from build123d import *

# Parameters (mm, degrees)
SKETCH1_W                                    = 107.95
SKETCH1_H                                    = 127
EXTRUDE1_DEPTH                               = 9.525
CBORE_FOR_M5_HEX_HEAD_CAP_SCREW2_D           = 5.5
CBORE_FOR_M5_HEX_HEAD_CAP_SCREW2_CBORE_D     = 12.24
CBORE_FOR_M5_HEX_HEAD_CAP_SCREW2_CBORE_DEPTH = 3.65
LPATTERN5_COUNT                              = 3
LPATTERN5_PITCH                              = 25.4
LPATTERN6_COUNT                              = 2
LPATTERN6_PITCH                              = 88.9
LPATTERN6_COPY_1_D                           = 5.5
LPATTERN6_COPY_1_CBORE_D                     = 12.24
LPATTERN6_COPY_1_CBORE_DEPTH                 = 3.65
LPATTERN6_COPY_2_D                           = 5.5
LPATTERN6_COPY_2_CBORE_D                     = 12.24
LPATTERN6_COPY_2_CBORE_DEPTH                 = 3.65
M5X0_8_TAPPED_HOLE1_D                        = 4.2
LPATTERN7_COUNT                              = 5
LPATTERN7_PITCH                              = 25.4
LPATTERN8_COUNT                              = 2
LPATTERN8_PITCH                              = 63.5
LPATTERN8_COPY_1_D                           = 4.2
LPATTERN8_COPY_2_D                           = 4.2
LPATTERN8_COPY_3_D                           = 4.2
LPATTERN8_COPY_4_D                           = 4.2
SKETCH16_W                                   = 107.95
SKETCH16_H                                   = 57.15
EXTRUDE2_DEPTH                               = 3.175


with BuildPart() as part:
    # Sketch1 → Extrude1 (new body)
    with BuildSketch(Plane.XY):
        Rectangle(SKETCH1_W, SKETCH1_H)
    extrude(amount=EXTRUDE1_DEPTH)

    # CBORE for M5 Hex Head Cap Screw2 (through all)
    with Locations(Plane(origin=(-44.45, -50.8, 9.525), x_dir=(1, 0, 0), z_dir=(0, 0, 1))):
        with Locations((0, 0)):
            cbore_for_m5_hex_head_cap_screw2 = CounterBoreHole(CBORE_FOR_M5_HEX_HEAD_CAP_SCREW2_D / 2, CBORE_FOR_M5_HEX_HEAD_CAP_SCREW2_CBORE_D / 2, CBORE_FOR_M5_HEX_HEAD_CAP_SCREW2_CBORE_DEPTH)

    # LPattern5: CBORE for M5 Hex Head Cap Screw2 ×3
    with Locations(*[(0, i * LPATTERN5_PITCH, 0) for i in range(1, LPATTERN5_COUNT)]):
        add(cbore_for_m5_hex_head_cap_screw2, mode=Mode.SUBTRACT)

    # LPattern6: CBORE for M5 Hex Head Cap Screw2 ×2
    with Locations(*[(i * LPATTERN6_PITCH, 0, 0) for i in range(1, LPATTERN6_COUNT)]):
        add(cbore_for_m5_hex_head_cap_screw2, mode=Mode.SUBTRACT)

    # LPattern6 copy 1 (through all)
    with Locations(Plane(origin=(44.45, -25.4, 9.525), x_dir=(1, 0, 0), z_dir=(0, 0, 1))):
        with Locations((0, 0)):
            CounterBoreHole(LPATTERN6_COPY_1_D / 2, LPATTERN6_COPY_1_CBORE_D / 2, LPATTERN6_COPY_1_CBORE_DEPTH)

    # LPattern6 copy 2 (through all)
    with Locations(Plane(origin=(44.45, 0, 9.525), x_dir=(1, 0, 0), z_dir=(0, 0, 1))):
        with Locations((0, 0)):
            CounterBoreHole(LPATTERN6_COPY_2_D / 2, LPATTERN6_COPY_2_CBORE_D / 2, LPATTERN6_COPY_2_CBORE_DEPTH)

    # M5x0.8 Tapped Hole1 (through all)
    with Locations(Plane(origin=(-31.75, -50.8, 9.525), x_dir=(1, 0, 0), z_dir=(0, 0, 1))):
        with Locations((0, 0)):
            m5x0_8_tapped_hole1 = Hole(M5X0_8_TAPPED_HOLE1_D / 2)

    # LPattern7: M5x0.8 Tapped Hole1 ×5
    with Locations(*[(0, i * LPATTERN7_PITCH, 0) for i in range(1, LPATTERN7_COUNT)]):
        add(m5x0_8_tapped_hole1, mode=Mode.SUBTRACT)

    # LPattern8: M5x0.8 Tapped Hole1 ×2
    with Locations(*[(i * LPATTERN8_PITCH, 0, 0) for i in range(1, LPATTERN8_COUNT)]):
        add(m5x0_8_tapped_hole1, mode=Mode.SUBTRACT)

    # LPattern8 copy 1 (through all)
    with Locations(Plane(origin=(31.75, -25.4, 9.525), x_dir=(1, 0, 0), z_dir=(0, 0, 1))):
        with Locations((0, 0)):
            Hole(LPATTERN8_COPY_1_D / 2)

    # LPattern8 copy 2 (through all)
    with Locations(Plane(origin=(31.75, 0, 9.525), x_dir=(1, 0, 0), z_dir=(0, 0, 1))):
        with Locations((0, 0)):
            Hole(LPATTERN8_COPY_2_D / 2)

    # LPattern8 copy 3 (through all)
    with Locations(Plane(origin=(31.75, 25.4, 9.525), x_dir=(1, 0, 0), z_dir=(0, 0, 1))):
        with Locations((0, 0)):
            Hole(LPATTERN8_COPY_3_D / 2)

    # LPattern8 copy 4 (through all)
    with Locations(Plane(origin=(31.75, 50.8, 9.525), x_dir=(1, 0, 0), z_dir=(0, 0, 1))):
        with Locations((0, 0)):
            Hole(LPATTERN8_COPY_4_D / 2)

    # Sketch16 → Extrude2 (cut)
    with BuildSketch(Plane(origin=(0, 0, 0), x_dir=(-1, 0, 0), z_dir=(0, 0, -1))):
        with Locations((0, 34.925)):
            Rectangle(SKETCH16_W, SKETCH16_H)
    extrude(amount=-EXTRUDE2_DEPTH, mode=Mode.SUBTRACT)


solid = part.part
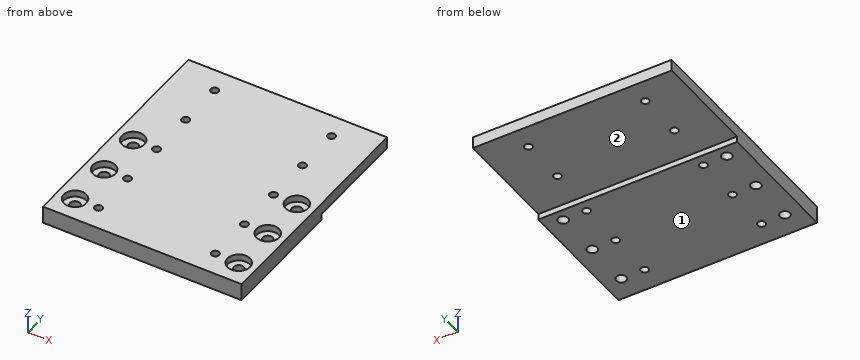
Read the model definition and answer for the solid it produces. Units are mm, in the model's axes. Face numbers are marked on the shaded views. A direction names the side the tool comes from. Coordinates: 2 decimals unless noted, no trailing zeros. Loops run counter-clockwise (first coordinate to the right, second up) from the corner with the lowest first, then second, coordinate; pieces in that order, holes last. Notation, with made-up numbers: (-32, 75) -> (-5, 75) arc R21 cw to (-5, 97) -> close; hole circle Ø9 at (75, -6.5). An arc over 180 degrees is marked (long way). Answer in a Markdown table with one row per item.
Item 1: A cutting plane is placed at B-B on y = 0. Determine the outline of the cut face in (x, z) (3 decimals).
Returned:
| item | result |
|---|---|
| outline | (-53.975, 0) -> (-47.2, 0) -> (-47.2, 5.875) -> (-50.57, 5.875) -> (-50.57, 9.525) -> (-53.975, 9.525) -> close; (-41.7, 0) -> (-33.85, 0) -> (-33.85, 9.525) -> (-38.33, 9.525) -> (-38.33, 5.875) -> (-41.7, 5.875) -> close; (-29.65, 0) -> (29.65, 0) -> (29.65, 9.525) -> (-29.65, 9.525) -> close; (33.85, 0) -> (41.7, 0) -> (41.7, 5.875) -> (38.33, 5.875) -> (38.33, 9.525) -> (33.85, 9.525) -> close; (47.2, 0) -> (53.975, 0) -> (53.975, 9.525) -> (50.57, 9.525) -> (50.57, 5.875) -> (47.2, 5.875) -> close |
Item 2: Each of these flat-tipped pins is pushed along its axis until it touches: P1, Ø3.5, axis at x = 31.75, y = -50.8, coming from the +Z side; P2, Ø1, axis at x = 13, z = 1, coming from the +Y side; P3, Ø11, axis at x = -44.45, y = -50.8, coming from the -Z side; P4, Ø3.5, axis at x = -44, y = -22.5, coming from the +Z side (3 decimals). Where does it stop, or does it pass through?
Returned:
| item | result |
|---|---|
| P1 | passes through |
| P2 | stops at y = 6.35 |
| P3 | stops at z = 0 |
| P4 | stops at z = 5.875 |
Item 3: For the marked faces 1 and 2, determine the directions among +Z, -Z, +X, -X, +Y, -Y from which every point of the face is accessible in a straight line to the end or side of a thin tool.
Returned:
| item | result |
|---|---|
| face 1 | -Z, +X, -X, +Y, -Y |
| face 2 | -Z, +X, -X, +Y |
Item 4: A cutting plane is placed at A-A on x = 44.45. Give the number of separate pieces and of enclosed holes in the cut face, plus the area to 3 significant figures.
Returned:
| item | result |
|---|---|
| separate pieces | 4 |
| enclosed holes | 0 |
| area | 797 mm^2 |
Item 5: A cutting plane is placed at C-C on x = -31.75. Determine the outline of the cut face in (y, z) (3 decimals).
Returned:
| item | result |
|---|---|
| outline | (-63.5, 0) -> (-52.9, 0) -> (-52.9, 9.525) -> (-63.5, 9.525) -> close; (-48.7, 0) -> (-27.5, 0) -> (-27.5, 9.525) -> (-48.7, 9.525) -> close; (-23.3, 0) -> (-2.1, 0) -> (-2.1, 9.525) -> (-23.3, 9.525) -> close; (2.1, 0) -> (6.35, 0) -> (6.35, 3.175) -> (23.3, 3.175) -> (23.3, 9.525) -> (2.1, 9.525) -> close; (27.5, 3.175) -> (48.7, 3.175) -> (48.7, 9.525) -> (27.5, 9.525) -> close; (52.9, 3.175) -> (63.5, 3.175) -> (63.5, 9.525) -> (52.9, 9.525) -> close |
Item 6: Straight lines are drawn through the part: line 1 along Y through (x, z) = (-44.45, 8.4); line 2 along Y through (x, z) = (-44.45, 1.85); line 3 along X through (y, z) = (-49, 9.25) (3 decimals). For each, find the intervals that lie inside material, in ascending order. Write a range as [from, to].
Returned:
| item | result |
|---|---|
| line 1 | y = [-63.5, -56.92], [-44.68, -31.52], [-19.28, -6.12], [6.12, 63.5] |
| line 2 | y = [-63.5, -53.55], [-48.05, -28.15], [-22.65, -2.75], [2.75, 6.35] |
| line 3 | x = [-53.975, -50.299], [-38.601, -32.832], [-30.668, 30.668], [32.832, 38.601], [50.299, 53.975] |
Item 7: A cutting plane is placed at D-D on y = 25.4. Determine the outline of the cut face in (x, z) (3 decimals), plus the area to 3 significant figures.
Returned:
| item | result |
|---|---|
| outline | (-53.975, 3.175) -> (-33.85, 3.175) -> (-33.85, 9.525) -> (-53.975, 9.525) -> close; (-29.65, 3.175) -> (29.65, 3.175) -> (29.65, 9.525) -> (-29.65, 9.525) -> close; (33.85, 3.175) -> (53.975, 3.175) -> (53.975, 9.525) -> (33.85, 9.525) -> close |
| area | 632 mm^2 |
